```python
from build123d import *

# Parameters (mm, degrees)
ESBO_O1_W                = 5
ESBO_O1_H                = 5.5
ESBO_O1_R                = 1.35
RESSALTO_EXTRUS_O1_DEPTH = 0.5
ESBO_O2_W                = 5
ESBO_O2_H                = 0.5
RESSALTO_EXTRUS_O2_DEPTH = 6.52
FILETE3_R                = 0.5
CORTE_EXTRUS_O1_DEPTH    = 9.973873188
CORTE_EXTRUS_O2_DEPTH    = 9.973873188
ESBO_O5_W                = 1
ESBO_O5_H                = 0.5
RESSALTO_EXTRUS_O3_DEPTH = 7.5
FILETE4_R                = 0.5
ESBO_O6_W                = 1.52
ESBO_O6_H                = 3
RESSALTO_EXTRUS_O4_DEPTH = 0.5
CORTE_EXTRUS_O3_DEPTH    = 13.672525399
FILETE4_OF_ESPELHAR2_R   = 0.5


with BuildPart() as part:
    # Esboço1 → Ressalto-extrusão1 (new body)
    with BuildSketch(Plane.XY):
        Rectangle(ESBO_O1_W, ESBO_O1_H)
        with Locations((0, 0.5)):
            Circle(ESBO_O1_R, mode=Mode.SUBTRACT)
    extrude(amount=-RESSALTO_EXTRUS_O1_DEPTH)

    # Esboço2 → Ressalto-extrusão2 (add)
    with BuildSketch(Plane(origin=(0, 0, -0.5), x_dir=(-1, 0, 0), z_dir=(0, 0, -1))):
        with Locations((0, -2.5)):
            Rectangle(ESBO_O2_W, ESBO_O2_H)
    extrude(amount=RESSALTO_EXTRUS_O2_DEPTH)

    # Filete3
    filete3_edges = [part.edges().sort_by_distance(p)[0] for p in [
        (0, -2.75, 0),
    ]]
    fillet(filete3_edges, radius=FILETE3_R)

    # Esboço3 → Corte-extrusão1 (cut, through all)
    with BuildSketch(Plane(origin=(0, -2.25, 0), x_dir=(1, 0, 0), z_dir=(0, 1, 0))):
        with BuildLine():
            Line((-0.5, 7.02), (-0.5, 3.52))
            ThreePointArc((-0.5, 3.52), (0, 3.02), (0.5, 3.52))
            Line((0.5, 3.52), (0.5, 7.02))
            Line((0.5, 7.02), (-0.5, 7.02))
        make_face()
    extrude(amount=-CORTE_EXTRUS_O1_DEPTH, mode=Mode.SUBTRACT)

    # Esboço4 → Corte-extrusão2 (cut, through all)
    with BuildSketch(Plane(origin=(0, -2.25, 0), x_dir=(1, 0, 0), z_dir=(0, 1, 0))):
        with BuildLine():
            Line((1.5, 7.02), (1.5, 3.52))
            ThreePointArc((1.5, 3.52), (2.207106781, 3.227106781), (2.5, 2.52))
            Line((2.5, 2.52), (2.5, 7.02))
            Line((2.5, 7.02), (1.5, 7.02))
        make_face()
    corte_extrus_o2 = extrude(amount=-CORTE_EXTRUS_O2_DEPTH, mode=Mode.SUBTRACT)

    # Espelhar1: Corte-extrusão2 across plane
    add(corte_extrus_o2.mirror(Plane(origin=(0, 0, 0), x_dir=(0, 0, 1), z_dir=(1, 0, 0))), mode=Mode.SUBTRACT)

    # Esboço5 → Ressalto-extrusão3 (add)
    with BuildSketch(Plane.XZ.offset(2.75)):
        with Locations((-1, -6.77)):
            Rectangle(ESBO_O5_W, ESBO_O5_H)
    ressalto_extrus_o3 = extrude(amount=RESSALTO_EXTRUS_O3_DEPTH)

    # Filete4
    filete4_edges = [part.edges().sort_by_distance(p)[0] for p in [
        (-1, -2.25, -7.02),
    ]]
    fillet(filete4_edges, radius=FILETE4_R)

    # Esboço6 → Ressalto-extrusão4 (add)
    with BuildSketch(Plane(origin=(0, 0, -7.02), x_dir=(-1, 0, 0), z_dir=(0, 0, -1))):
        with Locations((1.26, -8.75)):
            Rectangle(ESBO_O6_W, ESBO_O6_H)
    ressalto_extrus_o4 = extrude(amount=-RESSALTO_EXTRUS_O4_DEPTH)

    # Esboço7 → Corte-extrusão3 (cut, through all)
    with BuildSketch(Plane(origin=(0, 0, -7.02), x_dir=(-1, 0, 0), z_dir=(0, 0, -1))):
        with BuildLine():
            Line((1.5, -7.25), (2.02, -7.25))
            Line((2.02, -7.25), (2.02, -10.25))
            Line((2.02, -10.25), (0.5, -10.25))
            ThreePointArc((0.5, -10.25), (0.830266035, -10.152734868), (1.055096438, -9.891990837))
            Line((1.055096438, -9.891990837), (2, -7.805096438))
            ThreePointArc((2, -7.805096438), (1.691943399, -7.579842376), (1.5, -7.25))
        make_face()
    corte_extrus_o3 = extrude(amount=-CORTE_EXTRUS_O3_DEPTH, mode=Mode.SUBTRACT)

    # Espelhar2: Ressalto-extrusão3, Ressalto-extrusão4, Corte-extrusão3 across plane
    add(ressalto_extrus_o3.mirror(Plane(origin=(0, 0, 0), x_dir=(0, 0, 1), z_dir=(1, 0, 0))))
    add(ressalto_extrus_o4.mirror(Plane(origin=(0, 0, 0), x_dir=(0, 0, 1), z_dir=(1, 0, 0))))
    add(corte_extrus_o3.mirror(Plane(origin=(0, 0, 0), x_dir=(0, 0, 1), z_dir=(1, 0, 0))), mode=Mode.SUBTRACT)

    # Filete4 of Espelhar2
    filete4_of_espelhar2_edges = [part.edges().sort_by_distance(p)[0] for p in [
        (1, -2.25, -7.02),
    ]]
    fillet(filete4_of_espelhar2_edges, radius=FILETE4_OF_ESPELHAR2_R)


solid = part.part
```
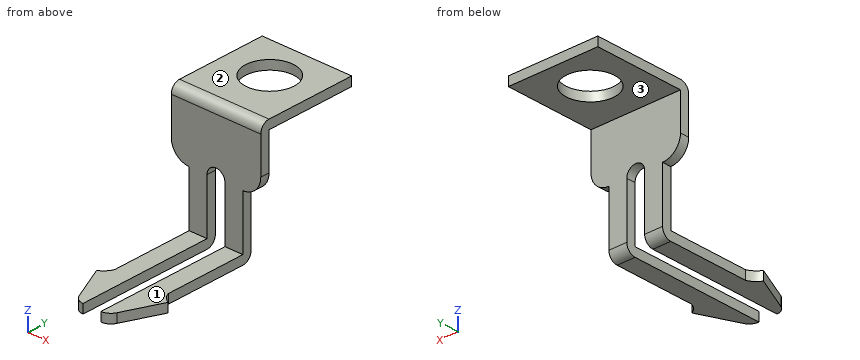
For this review, take the finished solid that the model builds, in its own axes (mm). Face numbers are marked on the shaded views. A direction names the side the tool comes from. Round coordinates to 2 decimals unless told otherwise and drop trailing zeros. Write each loop counter-clockwise with the first axis right and the second up, starting at its lowest first coordinate (ties: lowest second). Pieces come first, ordered by that corner, then holes. Notation, with made-up numbers: (74.25, 9.25) -> (83.25, 9.25) arc R20 cw to (83.25, 13.25) -> close; hole circle Ø10 at (64, -9.75). An arc over 180 degrees is marked (long way). One line per question, with ' | ' between items. Start each with the question number.
(1) For line 1 along Z through (x, y) = (1.1, -8.25); line 2 along Y through (x, z) = (0, -0.15); line 3 along Y through (x, z) = (0, -0.1), list the stretches that pass through material, from the lowest coordinate up. Write a range as from..to.
(2) Tool access review of the marked faces 1, 2 and 3: name each direction out of +Z, -Z, +X, -X, +Y, -Y from which nothing blocks a thin tool from reaching the whole face with its end or side.
(3) Add section B-B, the plane y = -5.5. Write out the cut boundary in (x, z).
(4) Add section C-C, the plane z = -5.25. Write out the cut boundary in (x, y), plus the area to 3 significant figures.
(5) Add section A-A, the plane x = 0. Write out the cut boundary in (y, z), plus the area to 3 significant figures.
(6) Insertion check: P1, Ø1, axis at x = -0.5, z = -5, coming from the -Y side; P2, Ø1.2, axis at x = -1.5, y = -8, coming from the +Z side; P3, Ø1, axis at x = -1, z = -2, coming from the +Y side. Each pin has a flat end and moves straight along its axis. Give the tip position at first contact, or say it passes through.
(7) Add section D-D, the plane x = -1.2. Write out the cut boundary in (y, z).
Answer list:
1) line 1: -7.02..-6.52 | line 2: -2.61..-0.85, 1.85..2.75 | line 3: -2.55..-0.85, 1.85..2.75
2) face 1: +Z, +X, -X, -Y | face 2: +Z, +X, -X, +Y, -Y | face 3: -Z, +X, -X, +Y
3) outline: (-1.5, -7.02) -> (-0.5, -7.02) -> (-0.5, -6.52) -> (-1.5, -6.52) -> close; (0.5, -7.02) -> (1.5, -7.02) -> (1.5, -6.52) -> (0.5, -6.52) -> close
4) outline: (-1.5, -2.75) -> (-0.5, -2.75) -> (-0.5, -2.25) -> (-1.5, -2.25) -> close; (0.5, -2.75) -> (1.5, -2.75) -> (1.5, -2.25) -> (0.5, -2.25) -> close | area: 1.00 mm²
5) outline: (-2.75, -3.02) -> (-2.25, -3.02) -> (-2.25, -0.5) -> (-0.85, -0.5) -> (-0.85, 0) -> (-2.25, 0) arc R0.5 ccw to (-2.75, -0.5) -> close; (1.85, -0.5) -> (2.75, -0.5) -> (2.75, 0) -> (1.85, 0) -> close | area: 2.61 mm²
6) P1: y = -2.75 | P2: z = -6.52 | P3: y = -2.25
7) outline: (-9.57, -7.02) -> (-2.75, -7.02) arc R0.5 ccw to (-2.25, -6.52) -> (-2.25, -0.5) -> (-0.12, -0.5) -> (-0.12, 0) -> (-2.25, 0) arc R0.5 ccw to (-2.75, -0.5) -> (-2.75, -6.52) -> (-9.57, -6.52) -> close; (1.12, -0.5) -> (2.75, -0.5) -> (2.75, 0) -> (1.12, 0) -> close
